```python
from build123d import *

# Parameters (mm, degrees)
F0_W     = 10
F0_H     = 5
F1_DEPTH = 40
F2_R     = 1
F3_DEPTH = 1
F4_R     = 1
F5_DEPTH = 1
F6_SIZE2 = 4.99999
F6_SIZE  = 9.99999


# Not quite as in the source:
# - a fillet or chamfer is up to 0.001 mm smaller than in the source, because OpenCascade refuses the exact size


with BuildPart() as f1:
    # F0 (on Front) → F1 (new body)
    with BuildSketch(Plane.XZ):
        Rectangle(F0_W, F0_H)
    extrude(amount=F1_DEPTH)

    # F2 (on face) → F3 (join)
    with BuildSketch(Plane.YZ.offset(5)):
        with BuildLine():
            Line((-24, 2.5), (-20, 2.5))
            ThreePointArc((-20, 2.5), (-24, 6.5), (-28, 2.5))
            Line((-28, 2.5), (-24, 2.5))
        make_face()
        with Locations((-24, 4.5)):
            Circle(F2_R, mode=Mode.SUBTRACT)
    extrude(amount=-F3_DEPTH)

    # F4 (on face) → F5 (join)
    with BuildSketch(Plane(origin=(-5, 0, 0), x_dir=(0, -1, 0), z_dir=(-1, 0, 0))):
        with BuildLine():
            ThreePointArc((28, 2.5), (24, 6.5), (20, 2.5))
            Line((20, 2.5), (24, 2.5))
            Line((24, 2.5), (28, 2.5))
        make_face()
        with Locations((24, 4.5)):
            Circle(F4_R, mode=Mode.SUBTRACT)
    extrude(amount=-F5_DEPTH)

    # F6 (size 10 and 5 in the source; OpenCascade refuses exactly that, so slightly less here)
    f6_edges = [f1.edges().sort_by_distance(p)[0] for p in [
        (0, -40, 2.5),
    ]]
    f6_side = f1.faces().sort_by_distance((0, -19.833333, 2.5))[0]
    chamfer(f6_edges, length=F6_SIZE, length2=F6_SIZE2, reference=f6_side)


solid = f1.part
```
Work out the finished part from the listing and answer in its coordinate system (mm). A direction names the side the tool comes from. Give positions to 0.01 mm unless a question says otherwise; leave off trailing zeros. Order: outer loops, then holes, each group sorted by start corner. A loop starts at its lowest first (then second) coordinate and runs counter-clockwise, first axis right, second up. Notation, with made-up numbers: (-7.75, -0.5) -> (45.25, -0.5) arc R13 ccw to (45.25, 14.5) -> close; hole circle Ø10 at (75.5, 61). An arc over 180 degrees is marked (long way). Answer as CSV lines item,"result". Start each with the question number.
(1) For a pull along Z with two mould halves and no side action, classify faces 1 (the cylindrical face through (-4.5, -24.1, 6.5)), 2 (the flat face through (0, -20, -2.5)), 3 (the cylindrical face through (4.507, -24.737, 5.176)) as released by +Z, released by -Z, zero draft, split by the parting line, or undercut.
(2) Section B-B, the plane z = 4.5 is taken. Write down the section's boundary in (x, y), plus the area to 3 significant figures.
(3) Section A-A, the plane y = -24 is taken. Write down the section's boundary in (x, z).
(4) Which of the six approach directions +Z, -Z, +X, -X, +Y, -Y give full straight-line access (tool end or side, diameter ignored) to faces 4 (the cylindrical face through (4.5, -23.9, 6.5)), 5 (the flat face through (4, -24, 3))?
(5) Consider line 1 along Z through (x, y) = (-4.25, -24); line 2 along Z through (x, y) = (-1.5, -25.5); line 3 along Y through (x, z) = (4.25, 4.25). Determine where each line is inside the solid, lowest interval first.
(6) Each of these flat-tipped pins is pushed along its axis until it touches: pin 1 Ø1 at (x, y) = (-1.5, -23) entering from +Z; pin 2 Ø4.5 at (y, z) = (-24, 4.5) entering from +X; pin 3 Ø1.8 at (y, z) = (-24, 4.5) entering from -X. Where does it stop, or does it pass through?
(7) Section D-D, the plane y = -30.5 is taken. Write down the section's boundary in (x, z).
Entries:
1,face 1,"released by +Z"
1,face 2,"released by -Z"
1,face 3,"undercut"
2,outline,"(-5, -27.46) -> (-4, -27.46) -> (-4, -25) -> (-5, -25) -> close; (-5, -23) -> (-4, -23) -> (-4, -20.54) -> (-5, -20.54) -> close; (4, -27.46) -> (5, -27.46) -> (5, -25) -> (4, -25) -> close; (4, -23) -> (5, -23) -> (5, -20.54) -> (4, -20.54) -> close"
2,area,"9.86 mm²"
3,outline,"(-5, -2.5) -> (5, -2.5) -> (5, 3.5) -> (4, 3.5) -> (4, 2.5) -> (-4, 2.5) -> (-4, 3.5) -> (-5, 3.5) -> close; (-5, 5.5) -> (-4, 5.5) -> (-4, 6.5) -> (-5, 6.5) -> close; (4, 5.5) -> (5, 5.5) -> (5, 6.5) -> (4, 6.5) -> close"
4,face 4,"+Z, +X, -X"
4,face 5,"+Z, +Y, -Y"
5,line 1,"-2.5 to 3.5, 5.5 to 6.5"
5,line 2,"-2.5 to 2.5"
5,line 3,"-27.6 to -24.97, -23.03 to -20.4"
6,pin 1,"z = 2.5"
6,pin 2,"x = 5"
6,pin 3,"through"
7,outline,"(-5, -2.5) -> (5, -2.5) -> (5, 2.25) -> (-5, 2.25) -> close"
